The listing builds one solid part. Answer for the finished solid, in the listing's coordinates (mm). A direction names the side the tool comes from. Round coordinates to 2 decimals unless told otherwise and drop trailing zeros. Write each loop counter-clockwise with the first axis right and the second up, starting at its lowest first coordinate (ties: lowest second). Pieces come first, ordered by that corner, then holes.
from build123d import *

# Parameters (mm, degrees)
SKETCH1_4_W                            = 360.68
SKETCH1_4_H                            = 132.08
SKETCH1_4_W_2                          = 27.94
SKETCH1_4_H_2                          = 93.98
BOSS_EXTRUDE3_DEPTH                    = 6.35
F_3_8_0_375_DIAMETER_HOLE1_D           = 9.525
F_3_8_0_375_DIAMETER_HOLE1_DEPTH       = 12.7
F_3_8_0_375_DIAMETER_HOLE1_CSINK_D     = 10.795
F_3_8_0_375_DIAMETER_HOLE1_CSINK_ANGLE = 90
F_3_8_0_375_DIAMETER_HOLE1_TIP         = 2.861598698
FILLET1_R                              = 12.7
SKETCH1_W                              = 27.94
SKETCH1_H                              = 93.98
BOSS_EXTRUDE4_DEPTH                    = 63.5
SKETCH10_R                             = 10.16
SKETCH10_R_2                           = 6.35
CUT_EXTRUDE11_DEPTH                    = 386.08
FILLET5_R                              = 6.35
F_1_2_0_5_DIAMETER_HOLE1_D             = 12.7
F_1_2_0_5_DIAMETER_HOLE1_DEPTH         = 13.97
F_1_2_0_5_DIAMETER_HOLE1_CSINK_D       = 13.97
F_1_2_0_5_DIAMETER_HOLE1_CSINK_ANGLE   = 90
F_1_2_0_5_DIAMETER_HOLE1_TIP           = 3.815464931
THREAD15_PITCH                         = 2.116666667
THREAD15_HEIGHT                        = 10
THREAD15_RADIUS                        = 10.16
THREAD15_START_ANGLE                   = -180
SKETCH25_W                             = 7.837170734
SKETCH25_H                             = 44.791396978
CUT_EXTRUDE12_DEPTH                    = 36.068
THREAD16_PITCH                         = 2.116666667
THREAD16_HEIGHT                        = 10
THREAD16_RADIUS                        = 10.16
THREAD16_START_ANGLE                   = -180
BOSS_EXTRUDE6_START                    = -15.24
SKETCH28_R                             = 10.16
BOSS_EXTRUDE6_DEPTH                    = 15.24
SKETCH29_R                             = 10.16
BOSS_EXTRUDE7_DEPTH                    = 15.24
SKETCH30_W                             = 15.24
SKETCH30_H                             = 93.98
CUT_EXTRUDE13_DEPTH                    = 57.15
SKETCH30_2_W                           = 15.24
SKETCH30_2_H                           = 93.98
CUT_EXTRUDE15_DEPTH                    = 139.954
SKETCH33_R                             = 6.35
CUT_EXTRUDE16_DEPTH                    = 343.916


with BuildPart() as part:
    # Sketch1<4> → Boss-Extrude3 (new body)
    with BuildSketch(Plane.XY):
        with Locations((180.34, 66.04)):
            Rectangle(SKETCH1_4_W, SKETCH1_4_H)
        with Locations((346.71, 66.04)):
            Rectangle(SKETCH1_4_W_2, SKETCH1_4_H_2)
    extrude(amount=-BOSS_EXTRUDE3_DEPTH)

    # 3/8 (0.375) Diameter Hole1
    with Locations(Plane.XY.offset(6.35)):
        with Locations((187.96, 124.46), (285.75, 124.46), (90.17, 124.46), (90.17, 7.62), (187.96, 7.62), (285.75, 7.62)):
            CounterSinkHole(F_3_8_0_375_DIAMETER_HOLE1_D / 2, F_3_8_0_375_DIAMETER_HOLE1_CSINK_D / 2, depth=F_3_8_0_375_DIAMETER_HOLE1_DEPTH, counter_sink_angle=F_3_8_0_375_DIAMETER_HOLE1_CSINK_ANGLE)
            with Locations((0, 0, -(F_3_8_0_375_DIAMETER_HOLE1_DEPTH + F_3_8_0_375_DIAMETER_HOLE1_TIP / 2))):  # 118° drill point
                Cone(0, F_3_8_0_375_DIAMETER_HOLE1_D / 2, F_3_8_0_375_DIAMETER_HOLE1_TIP, mode=Mode.SUBTRACT)

    # Fillet1
    fillet1_edges = [part.edges().sort_by_distance(p)[0] for p in [
        (0, 0, -3.175),
        (0, 132.08, -3.175),
        (360.68, 132.08, -3.175),
        (360.68, 0, -3.175),
    ]]
    fillet(fillet1_edges, radius=FILLET1_R)

    # Sketch1 → Boss-Extrude4 (add)
    with BuildSketch(Plane.XY):
        with Locations((346.71, 66.04)):
            Rectangle(SKETCH1_W, SKETCH1_H)
        with Locations((13.97, 66.04)):
            Rectangle(SKETCH1_W, SKETCH1_H)
    extrude(amount=-BOSS_EXTRUDE4_DEPTH)

    # Sketch10 → Cut-Extrude11 (cut)
    with BuildSketch(Plane(origin=(360.68, 0, 0), x_dir=(0, 0, -1), z_dir=(1, 0, 0))):
        with Locations((45.72, 66.04)):
            Circle(SKETCH10_R)
        with Locations((25.4, 66.04)):
            Circle(SKETCH10_R_2)
    extrude(amount=-CUT_EXTRUDE11_DEPTH, mode=Mode.SUBTRACT)

    # Fillet5
    fillet5_edges = [part.edges().sort_by_distance(p)[0] for p in [
        (360.68, 113.03, -34.925),
        (360.68, 66.04, -63.5),
        (360.68, 19.05, -34.925),
        (0, 113.03, -34.925),
        (0, 19.05, -34.925),
        (0, 66.04, -63.5),
    ]]
    fillet(fillet5_edges, radius=FILLET5_R)

    # 1/2 (0.5) Diameter Hole1
    with Locations(Plane.XY):
        with Locations((208.28, 66.04), (81.28, 66.04), (53.34, 66.04), (307.34, 66.04)):
            CounterSinkHole(F_1_2_0_5_DIAMETER_HOLE1_D / 2, F_1_2_0_5_DIAMETER_HOLE1_CSINK_D / 2, depth=F_1_2_0_5_DIAMETER_HOLE1_DEPTH, counter_sink_angle=F_1_2_0_5_DIAMETER_HOLE1_CSINK_ANGLE)
            with Locations((0, 0, -(F_1_2_0_5_DIAMETER_HOLE1_DEPTH + F_1_2_0_5_DIAMETER_HOLE1_TIP / 2))):  # 118° drill point
                Cone(0, F_1_2_0_5_DIAMETER_HOLE1_D / 2, F_1_2_0_5_DIAMETER_HOLE1_TIP, mode=Mode.SUBTRACT)

    # Thread15: sweep along a helix
    with BuildLine() as thread15_path:
        add(Helix(THREAD15_PITCH, THREAD15_HEIGHT, THREAD15_RADIUS, center=(360.68, 66.04, -45.72), direction=(-1, 0, 0), mode=Mode.PRIVATE).rotate(Axis((360.68, 66.04, -45.72), (-1, 0, 0)), THREAD15_START_ANGLE))
    # Thread Profile13 → Thread15 (sweep)
    with BuildSketch(Plane(origin=(360.68, 66.04, -35.56), x_dir=(0, 0, 1), z_dir=(0, -1, 0))):
        Polygon((0, 0), (0, 1.852083328), (-1.145679435, 1.190624997), (-1.145679435, 0.66145833), align=None)
    sweep(path=thread15_path.line, is_frenet=True)

    # Sketch25 → Cut-Extrude12 (cut)
    with BuildSketch(Plane(origin=(0, 0, -6.35), x_dir=(-1, 0, 0), z_dir=(0, 0, -1))):
        with Locations((-322.656094919, 66.002101848)):
            Rectangle(SKETCH25_W, SKETCH25_H)
    extrude(amount=-CUT_EXTRUDE12_DEPTH, mode=Mode.SUBTRACT)

    # Thread16: sweep along a helix
    with BuildLine() as thread16_path:
        add(Helix(THREAD16_PITCH, THREAD16_HEIGHT, THREAD16_RADIUS, center=(0, 66.04, -45.72), direction=(1, 0, 0), mode=Mode.PRIVATE).rotate(Axis((0, 66.04, -45.72), (1, 0, 0)), THREAD16_START_ANGLE))
    # Thread Profile14 → Thread16 (sweep, cut)
    with BuildSketch(Plane(origin=(0, 66.04, -55.88), x_dir=(0, 0, -1), z_dir=(0, -1, 0))):
        Polygon((0, 0), (0, 1.852083328), (-1.145679435, 1.190624997), (-1.145679435, 0.66145833), align=None)
    sweep(path=thread16_path.line, is_frenet=True, mode=Mode.SUBTRACT)

    # Sketch28 → Boss-Extrude6 (add)
    with BuildSketch(Plane.ZY.offset(-332.74).offset(BOSS_EXTRUDE6_START)):
        with Locations((-45.72, 66.04)):
            Circle(SKETCH28_R)
    extrude(amount=BOSS_EXTRUDE6_DEPTH)

    # Sketch29 → Boss-Extrude7 (add)
    with BuildSketch(Plane(origin=(27.94, 0, 0), x_dir=(0, 0, -1), z_dir=(1, 0, 0))):
        with Locations((45.72, 66.04)):
            Circle(SKETCH29_R)
    extrude(amount=-BOSS_EXTRUDE7_DEPTH)

    # Sketch30 → Cut-Extrude13 (cut)
    with BuildSketch(Plane(origin=(0, 0, -63.5), x_dir=(-1, 0, 0), z_dir=(0, 0, -1))):
        with Locations((-353.06, 66.04)):
            Rectangle(SKETCH30_W, SKETCH30_H)
        with Locations((-7.62, 66.04)):
            Rectangle(SKETCH30_W, SKETCH30_H)
    extrude(amount=-CUT_EXTRUDE13_DEPTH, mode=Mode.SUBTRACT)

    # Sketch30<2> → Cut-Extrude15 (cut)
    with BuildSketch(Plane(origin=(0, 0, -63.5), x_dir=(-1, 0, 0), z_dir=(0, 0, -1))):
        with Locations((-353.06, 66.04)):
            Rectangle(SKETCH30_2_W, SKETCH30_2_H)
        with Locations((-7.62, 66.04)):
            Rectangle(SKETCH30_2_W, SKETCH30_2_H)
    extrude(amount=-CUT_EXTRUDE15_DEPTH, mode=Mode.SUBTRACT)

    # Sketch33 → Cut-Extrude16 (cut)
    with BuildSketch(Plane(origin=(345.44, 0, 0), x_dir=(0, 0, -1), z_dir=(1, 0, 0))):
        with Locations(Location((45.72, 66.04, 0), (0, 0, 90))):
            Circle(SKETCH33_R)
    extrude(amount=-CUT_EXTRUDE16_DEPTH, mode=Mode.SUBTRACT)


solid = part.part
1. For a pull along Y with two mould halves and no side action, classify faces 4 (the face through (357.06, 3.82, -3.22)), 5 (the face through (290.508, 124.669, -3.219)), 6 (the face through (0, 116, -3)) as released by +Y, released by -Y, zero draft, split by the parting line, or undercut.
Geometry says:
face 4: released by -Y
face 5: undercut
face 6: zero draft
2. Section A-A on z = -10 is taken. Determine the outline of the cut face in (x, y), plus the area to 3 significant figures.
Geometry says:
outline: (15.24, 19.05) - (27.94, 19.05) - (27.94, 113.03) - (15.24, 113.03) - close; (332.74, 19.05) - (345.44, 19.05) - (345.44, 113.03) - (332.74, 113.03) - close
area: 2,390 mm2
3. Section C-C on x = 53.34 is taken. Determine the outline of the cut face in (y, z) (3 decimals), plus the area to 3 significant figures.
Geometry says:
outline: (0, -6.35) - (59.69, -6.35) - (59.69, -0.635) - (59.055, 0) - (0, 0) - close; (72.39, -6.35) - (132.08, -6.35) - (132.08, 0) - (73.025, 0) - (72.39, -0.635) - close
area: 758 mm2
4. Section B-B on y = 109.5 is taken. Determine the outline of the cut face in (x, z).
Geometry says:
outline: (15.24, -63.5) - (27.94, -63.5) - (27.94, -6.35) - (332.74, -6.35) - (332.74, -63.5) - (345.44, -63.5) - (345.44, 0) - (15.24, 0) - close
5. Straight lines are drawn through the part: line 1 along X through (y, z) = (66.04, -5.1); line 2 along Y through (x, z) = (285.75, -1.5); line 3 along Z through (x, y) = (25, 66). For each, find the intervals that lie inside material, in ascending order.
Geometry says:
line 1: x = 15.24 to 46.99, 59.69 to 74.93, 87.63 to 201.93, 214.63 to 300.99, 313.69 to 318.74, 326.57 to 345.44
line 2: y = 0 to 2.86, 12.38 to 119.7, 129.22 to 132.08
line 3: z = -63.5 to -52.07, -39.37 to -31.75, -19.05 to 0
6. A tool of negligible diameter and unlimited length cuts with its end or side. For faces 1 (the face through (22, 19.05, -35)), 2 (the face through (323, 43.606, -3)), 3 (the face through (353, 113.03, -3)), from which of +Z, -Z, +X, -X, +Y, -Y can it reach the whole face along a straight path? Write none if from no direction.
Geometry says:
face 1: -Z, +X, -X, -Y
face 2: +Z, -Z
face 3: +Z, -Z, +X
7. Given pin 1 (10 mm diameter, centred on y = 117.5, z = -51.5, fed in from +X); pin 2 (6.5 mm diameter, centred on x = 340, z = -25.5, fed in from -Y); pin 3 (8.5 mm diameter, centred on x = 90.17, y = 124.46, fed in from +Z); pin 4 (1.9 mm diameter, centred on x = 5.5, z = -3, fed in from +Y), each flat-ended and moving along its own axis, determine where each tip first touches the part or whether it passes through.
Geometry says:
pin 1: stops at x = 345.44
pin 2: stops at y = 19.05
pin 3: passes through
pin 4: stops at y = 130.44
8. Section D-D on y = 7.62 is taken. Determine the outline of the cut face in (x, z), plus the area to 3 significant figures.
Geometry says:
outline: (1.06, -6.35) - (85.41, -6.35) - (85.41, 0) - (1.06, 0) - close; (94.93, -6.35) - (183.2, -6.35) - (183.2, 0) - (94.93, 0) - close; (192.72, -6.35) - (280.99, -6.35) - (280.99, 0) - (192.72, 0) - close; (290.51, -6.35) - (359.62, -6.35) - (359.62, 0) - (290.51, 0) - close
area: 2,100 mm2
